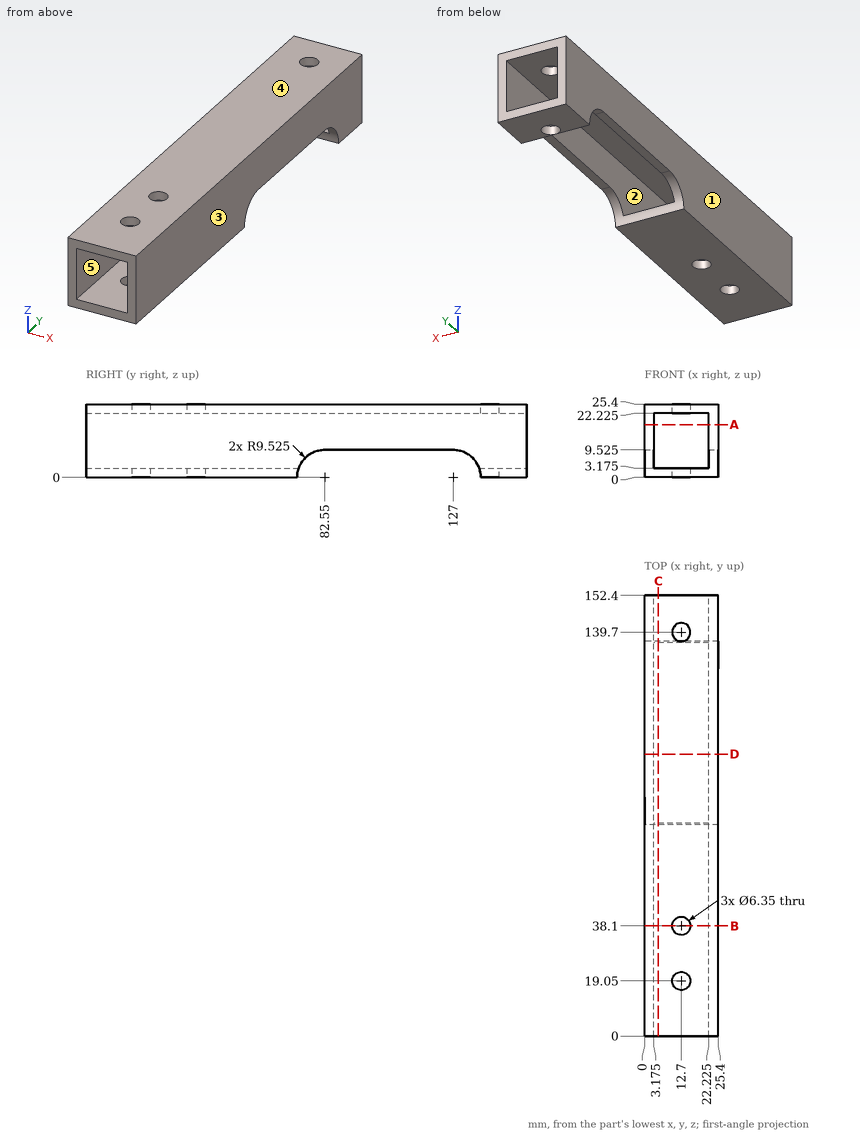
Geometry: see drawing. Coordinates: mm, zero at the bounding-box minimum. A direction names the side the tool comes from. Round coordinates to 2 decimals unless told otherwise and drop trailing zeros. Loops run counter-clockwise (first coordinate to the right, second up) from the corner with the lowest first, then second, coordinate; pieces in that order, holes last. Notation, with made-up numbers: M -39,-40 L -18,-40 A36 cw -18,-3 Z; hole C -24,37.5 d6. An arc over 180 degrees is marked long. Use a Markdown table: item, result. Add a question column.
1. Cut plane C-C, the plane x = 4.75. Output: boundary loops of the cut face in (y, z) (3 decimals).
2. Contact query for flat-ended pins moving along their axis: pin 1 (4 mm diameter, centred on x = 5.5, z = 11, fed in from +Y); pin 2 (1 mm diameter, centred on x = 2, y = 99.5, fed in from -Z) (3 decimals); pin 3 (5 mm diameter, centred on x = 11, y = 89, fed in from -Z) (3 decimals). Output: stop coordinate, or through.
3. Cut plane B-B, the plane y = 38.1. Output: boundary loops of the cut face in (x, z) (3 decimals), and give its area (3 significant figures).
4. Cut plane A-A, the plane z = 18.25. Output: boundary loops of the cut face in (x, y) (3 decimals).
5. Pull-direction query (Z, two-part tool) for the marked faces 3, 4 and 5; classes: +Z half, -Z half, draft (parallel to the pull), parting line (faces both ways), or undercut.
6. Cut plane D-D, the plane y = 97.5. Output: boundary loops of the cut face in (x, z) (3 decimals).
7. Ray query, line 1 along Y through (x, z) = (12.7, 23.3) (3 decimals); line 2 along Z through (x, y) = (5.5, 27.5) (3 decimals). Return the intervals inside material, ascending. Write a range as [from, to].
8. Set-up query: the marked faces 1 and 2. Return all of +Z, -Z, +X, -X, +Y, -Y with unobstructed straight access to the full face (end or side cutting, diameter ignored); none if empty.
Solution:
| question | item | result |
|---|---|---|
| 1 | outline | M 0,0 L 73.025,0 A9.525 cw 73.57,3.175 L 0,3.175 Z; M 0,22.225 L 152.4,22.225 L 152.4,25.4 L 0,25.4 Z; M 135.98,3.175 A9.525 cw 136.525,0 L 152.4,0 L 152.4,3.175 Z |
| 2 | pin 1 | passes through |
| 2 | pin 2 | stops at z = 9.525 |
| 2 | pin 3 | stops at z = 22.225 |
| 3 | outline | M 0,0 L 9.525,0 L 9.525,3.175 L 3.175,3.175 L 3.175,22.225 L 9.525,22.225 L 9.525,25.4 L 0,25.4 Z; M 15.875,0 L 25.4,0 L 25.4,25.4 L 15.875,25.4 L 15.875,22.225 L 22.225,22.225 L 22.225,3.175 L 15.875,3.175 Z |
| 3 | area | 242 mm2 |
| 4 | outline | M 0,0 L 3.175,0 L 3.175,152.4 L 0,152.4 Z; M 22.225,0 L 25.4,0 L 25.4,152.4 L 22.225,152.4 Z |
| 5 | face 3 | draft |
| 5 | face 4 | +Z half |
| 5 | face 5 | undercut |
| 6 | outline | M 0,9.525 L 3.175,9.525 L 3.175,22.225 L 22.225,22.225 L 22.225,9.525 L 25.4,9.525 L 25.4,25.4 L 0,25.4 Z |
| 7 | line 1 | y = [0, 15.875], [22.225, 34.925], [41.275, 136.525], [142.875, 152.4] |
| 7 | line 2 | z = [0, 3.175], [22.225, 25.4] |
| 8 | face 1 | +Z, -Z, -X, +Y, -Y |
| 8 | face 2 | +Y, -Y |
